from build123d import *

# Parameters (mm, degrees)
F0_R     = 1.6706088
F0_R_2   = 1.1185144
F0_R_3   = 1.0956036
F1_DEPTH = 1.5748


# Not quite as in the source:
# - ends of sketch curves that miss each other by under 0.0002 mm in the source are joined


with BuildPart() as f1:
    # F0 (on Top) → F1 (new body)
    with BuildSketch(Plane.XY):
        with BuildLine():
            Line((-23.2852722, 11.6233956), (-25.6565654, 11.6233956))
            Line((-25.6565654, 11.6233956), (-28.0302208, 11.6233956))
            ThreePointArc((-28.0302208, 11.6233956), (-29.0641368167, 11.2522249645), (-29.6259080683, 10.3082106474))
            Line((-29.6259080683, 10.3082106474), (-31.944437, -1.6106394))
            ThreePointArc((-31.944437, -1.6106394), (-31.2390678474, -5.2827981728), (-28.1896575043, -7.446928172))
            Line((-28.1896575043, -7.446928172), (-10.768076, -11.623421))
            Line((-10.768076, -11.623421), (0, -11.623421))
            Line((0, -11.623421), (10.768076, -11.623421))
            Line((10.768076, -11.623421), (28.1896566, -7.4469244))
            ThreePointArc((28.1896566, -7.4469244), (31.2390678474, -5.2827981728), (31.9444603849, -1.610634851))
            Line((31.9444603849, -1.610634851), (29.6258996, 10.308209))
            ThreePointArc((29.6258996, 10.308209), (29.0641368167, 11.2522249645), (28.0302208, 11.6233956))
            Line((28.0302208, 11.6233956), (25.6565654, 11.6233956))
            Line((25.6565654, 11.6233956), (23.2852722, 11.6233956))
            ThreePointArc((23.2852722, 11.6233956), (22.1357994165, 11.1472683835), (21.6596722, 9.9977956))
            Line((21.6596722, 9.9977956), (21.6596722, 2.2361652))
            ThreePointArc((21.6596722, 2.2361652), (21.4216085917, 1.6614288083), (20.8468722, 1.4233652))
            Line((20.8468722, 1.4233652), (0, 1.4233652))
            Line((0, 1.4233652), (-20.8468722, 1.4233652))
            ThreePointArc((-20.8468722, 1.4233652), (-21.4216085917, 1.6614288083), (-21.6596722, 2.2361652))
            Line((-21.6596722, 2.2361652), (-21.6596722, 9.9977956))
            ThreePointArc((-21.6596722, 9.9977956), (-22.1357994165, 11.1472683835), (-23.2852722, 11.6233956))
        make_face()
        with Locations((-27.0201644, -2.5685496)):
            Circle(F0_R, mode=Mode.SUBTRACT)
        with Locations((-6.7222878, -4.3003216)):
            Circle(F0_R_2, mode=Mode.SUBTRACT)
        with Locations((6.7222878, -4.3003216)):
            Circle(F0_R_2, mode=Mode.SUBTRACT)
        with Locations((27.0201644, -2.5685496)):
            Circle(F0_R, mode=Mode.SUBTRACT)
        with Locations((-25.658445, 8.6478872)):
            Circle(F0_R_3, mode=Mode.SUBTRACT)
        with Locations((25.658445, 8.6478872)):
            Circle(F0_R_3, mode=Mode.SUBTRACT)
    extrude(amount=F1_DEPTH)


solid = f1.part
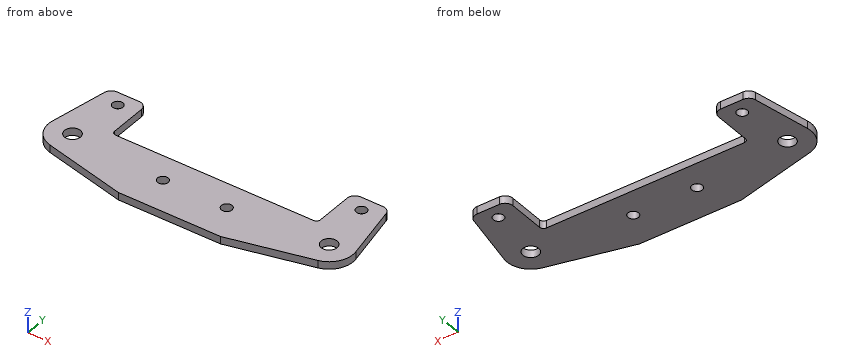
Verification items for the finished model (mm, model axes). Round coordinates to 2 decimals unless told otherwise and drop trailing zeros. Write each loop counter-clockwise with the first axis right and the second up, starting at its lowest first coordinate (ties: lowest second). Pieces come first, ordered by that corner, then holes.
(1) Section check B-B (y = 5). Enter the section's corners in (x, z), plus the area to 3 significant figures.
Returned:
outline: (-30.66, 0) - (-21.66, 0) - (-21.66, 1.57) - (-30.66, 1.57) - close; (21.66, 0) - (30.66, 0) - (30.66, 1.57) - (21.66, 1.57) - close
area: 28.3 mm2
(2) Section check A-A (x = -6.5). Enter the section's corners in (y, z), plus the area to 3 significant figures.
Returned:
outline: (-11.62, 0) - (-5.4, 0) - (-5.4, 1.57) - (-11.62, 1.57) - close; (-3.2, 0) - (1.42, 0) - (1.42, 1.57) - (-3.2, 1.57) - close
area: 17.1 mm2
(3) Section check D-D (x = 1). Enter the section's corners in (y, z), plus the area to 3 significant figures.
Returned:
outline: (-11.62, 0) - (1.42, 0) - (1.42, 1.57) - (-11.62, 1.57) - close
area: 20.5 mm2
(4) Section check C-C (z = 1.25). Enter the section's corners in (x, y).
Returned:
outline: (-31.94, -1.61) arc R5.02 ccw to (-28.19, -7.45) - (-10.77, -11.62) - (10.77, -11.62) - (28.19, -7.45) arc R5.02 ccw to (31.94, -1.61) - (29.63, 10.31) arc R1.63 ccw to (28.03, 11.62) - (23.29, 11.62) arc R1.63 ccw to (21.66, 10) - (21.66, 2.24) arc R0.81 cw to (20.85, 1.42) - (-20.85, 1.42) arc R0.81 cw to (-21.66, 2.24) - (-21.66, 10) arc R1.63 ccw to (-23.29, 11.62) - (-28.03, 11.62) arc R1.63 ccw to (-29.63, 10.31) - close; hole circle Ø3.34 at (-27.02, -2.57); hole circle Ø2.19 at (-25.66, 8.65); hole circle Ø2.24 at (-6.72, -4.3); hole circle Ø2.24 at (6.72, -4.3); hole circle Ø2.19 at (25.66, 8.65); hole circle Ø3.34 at (27.02, -2.57)
(5) Material ranges on line 1 (X direction, y = 2, z = 0.15); line 2 (X direction, y = 5.75, z = 1.4); line 3 (X direction, y = 8, z = 1.2), recorded low to high.
Returned:
line 1: x = -31.24 to -21.62, 21.62 to 31.24
line 2: x = -30.51 to -21.66, 21.66 to 30.51
line 3: x = -30.07 to -26.54, -24.77 to -21.66, 21.66 to 24.77, 26.54 to 30.07
